Design review of the part built by this model. Coordinates are the model's own, in mm. Face numbers are marked on the shaded views. A direction names the side the tool comes from. Coordinates: 2 decimals unless noted, no trailing zeros. Loops run counter-clockwise (first coordinate to the right, second up) from the corner with the lowest first, then second, coordinate; pieces in that order, holes last.
Q1. Add section C-C on z = 24. Give the boundary of the cut face in (x, y), and give its area (3 significant figures).
Q2. Wall thickness on probe 1 along Z at (x, y) = (-12.5, -15); probe 2 along Z at (x, y) = (22, -31); probe 3 along X at (y, z) = (-39, 35.5): over which ranges is each line inside the solid? List them lowest first.
Q3. Add section B-B on x = -2.5. Give the boundary of the cut face in (y, z).
Q4. Add section D-D on x = -22. Give the boundary of the cut face in (y, z).
Q5. Draft analysis for pull direction X (two halves, no side actions). For the marked faces 1, 2 and 3, state which applies: released by +X, released by -X, zero draft, split by the parting line, or undercut.
Q6. Machinability: for the marked faces 4, 5, 6, 7 and 8, which of the approach directions +Z, -Z, +X, -X, +Y, -Y give a long, thin tool a straight path to every point of the face, cutting with its end or side? Answer none if there is none.
Q7. Add section A-A on y = -34. Give the boundary of the cut face in (x, z).
Q8. For P1, Ø12, axis at x = -19, y = -40, coming from the -Z side; P2, Ø12, axis at x = 17, y = -26, coming from the +Z side; P3, Ø7.5, axis at x = -6, z = 13.5, coming from the -Y side; P4, Ø4, axis at x = -29.5, z = 30.5, coming from the -Y side, all flat-tipped, find the tip position at first contact; note any pin that passes through.
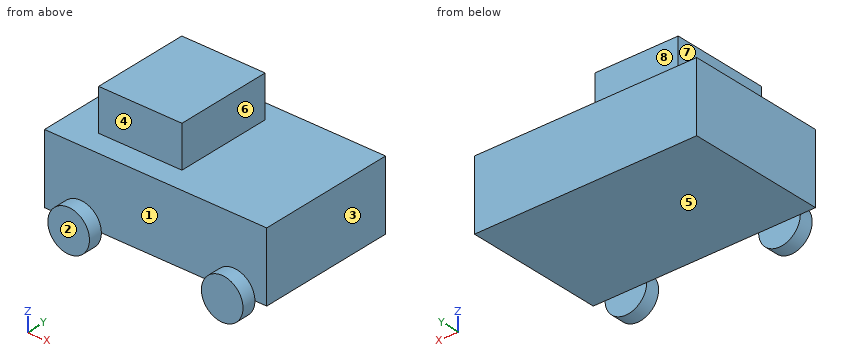
```python
from build123d import *

# Parameters (mm, degrees)
F0_W     = 80
F0_H     = 50
F1_DEPTH = 25
F2_W     = 30
F2_H     = 35
F3_DEPTH = 15
F5_DEPTH = 5


with BuildPart() as f1:
    # F0 (on Top) → F1 (new body)
    with BuildSketch(Plane.XY):
        with Locations((0.632411, -25)):
            Rectangle(F0_W, F0_H)
    extrude(amount=F1_DEPTH)

    # F2 (on face) → F3 (join)
    with BuildSketch(Plane.XY.offset(25)):
        with Locations((-11.804453, -24.404109)):
            Rectangle(F2_W, F2_H)
    extrude(amount=F3_DEPTH)

    # F4 (on face) → F5 (join)
    with BuildSketch(Plane.XZ.offset(50)):
        with BuildLine():
            Line((-33.882271, 0), (-18.882271, 0))
            ThreePointArc((-18.882271, 0), (-26.382271, 7.5), (-33.882271, 0))
        make_face()
        with BuildLine():
            Line((36.384543, 0), (21.384543, 0))
            ThreePointArc((21.384543, 0), (28.884543, -7.5), (36.384543, 0))
        make_face()
        with BuildLine():
            ThreePointArc((-33.882271, 0), (-26.382271, -7.5), (-18.882271, 0))
            Line((-18.882271, 0), (-33.882271, 0))
        make_face()
        with BuildLine():
            ThreePointArc((36.384543, 0), (28.884543, 7.5), (21.384543, 0))
            Line((21.384543, 0), (36.384543, 0))
        make_face()
    extrude(amount=F5_DEPTH)


solid = f1.part
```
Entries:
1. outline: (-39.37, -50) - (40.63, -50) - (40.63, 0) - (-39.37, 0) - close
1. area: 4,000 mm2
2. probe 1: z = 0 to 40
2. probe 2: z = 0 to 25
2. probe 3: x = -26.8 to 3.2
3. outline: (-50, 0) - (0, 0) - (0, 25) - (-6.9, 25) - (-6.9, 40) - (-41.9, 40) - (-41.9, 25) - (-50, 25) - close
4. outline: (-55, -6.09) - (-50, -6.09) - (-50, 0) - (0, 0) - (0, 25) - (-6.9, 25) - (-6.9, 40) - (-41.9, 40) - (-41.9, 25) - (-50, 25) - (-50, 6.09) - (-55, 6.09) - close
5. face 1: undercut
5. face 2: zero draft
5. face 3: released by +X
6. face 4: +Z, +X, -X, -Y
6. face 5: -Z, +X, -X, +Y
6. face 6: +Z, +X, +Y, -Y
6. face 7: +Z, -X, +Y, -Y
6. face 8: +Z, +X, -X, +Y
7. outline: (-39.37, 0) - (40.63, 0) - (40.63, 25) - (3.2, 25) - (3.2, 40) - (-26.8, 40) - (-26.8, 25) - (-39.37, 25) - close
8. P1: stops at z = 0
8. P2: stops at z = 25
8. P3: stops at y = -50
8. P4: passes through
